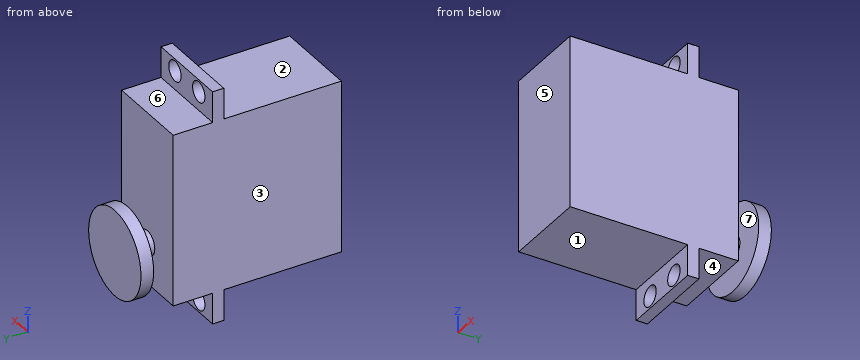
```python
from build123d import *

# Parameters (mm, degrees)
SKETCH1_W           = 19.8
SKETCH1_H           = 40.15
BOSS_EXTRUDE1_DEPTH = 39.2
SKETCH4_W           = 19.8
SKETCH4_H           = 2.6
BOSS_EXTRUDE2_DEPTH = 7.225
CUT_EXTRUDE1_REACH  = 43.753
SKETCH5_R           = 2.375
SKETCH6_R           = 2.825
BOSS_EXTRUDE3_DEPTH = 4.65
SKETCH8_R           = 10.05
BOSS_EXTRUDE4_DEPTH = 2.95


with BuildPart() as part:
    # Sketch1 → Boss-Extrude1 (new body)
    with BuildSketch(Plane(origin=(0, 0, 0), x_dir=(1, 0, 0), z_dir=(0, 1, 0))):
        Rectangle(SKETCH1_W, SKETCH1_H)
    extrude(amount=BOSS_EXTRUDE1_DEPTH)

    # Sketch4 → Boss-Extrude2 (add)
    with BuildSketch(Plane(origin=(0, 0, -20.075), x_dir=(-1, 0, 0), z_dir=(0, 0, -1))):
        with Locations((0, 28.7)):
            Rectangle(SKETCH4_W, SKETCH4_H)
    boss_extrude2 = extrude(amount=BOSS_EXTRUDE2_DEPTH)

    # Sketch5 → Cut-Extrude1 (cut, up to next)
    with BuildSketch(Plane(origin=(0, 30, 0), x_dir=(1, 0, 0), z_dir=(0, 1, 0)), mode=Mode.PRIVATE) as cut_extrude1_sk1:
        with Locations(Location((4.575, 24.45, 0), (0, 0, 270))):
            Circle(SKETCH5_R)
    cut_extrude1_tool1 = extrude(cut_extrude1_sk1.sketch, amount=-CUT_EXTRUDE1_REACH, mode=Mode.PRIVATE) & part.part
    # Sketch5 → Cut-Extrude1 (cut, up to next)
    with BuildSketch(Plane(origin=(0, 30, 0), x_dir=(1, 0, 0), z_dir=(0, 1, 0)), mode=Mode.PRIVATE) as cut_extrude1_sk2:
        with Locations(Location((-4.575, 24.45, 0), (0, 0, 270))):
            Circle(SKETCH5_R)
    cut_extrude1_tool2 = extrude(cut_extrude1_sk2.sketch, amount=-CUT_EXTRUDE1_REACH, mode=Mode.PRIVATE) & part.part
    cut_extrude1_1 = cut_extrude1_tool1.solids().sort_by_distance((4.575, 30, -24.45))[0]
    add(cut_extrude1_1, mode=Mode.SUBTRACT)
    cut_extrude1_2 = cut_extrude1_tool2.solids().sort_by_distance((-4.575, 30, -24.45))[0]
    add(cut_extrude1_2, mode=Mode.SUBTRACT)
    cut_extrude1 = cut_extrude1_1 + cut_extrude1_2  # Cut-Extrude1 as one shape, for the pattern or mirror that repeats it

    # Mirror2: Boss-Extrude2, Cut-Extrude1 across plane
    add(boss_extrude2.mirror(Plane.XY))
    add(cut_extrude1.mirror(Plane.XY), mode=Mode.SUBTRACT)

    # Sketch6 → Boss-Extrude3 (add)
    with BuildSketch(Plane(origin=(0, 39.2, 0), x_dir=(1, 0, 0), z_dir=(0, 1, 0))):
        with Locations(Location((0, 10.475, 0), (0, 0, 270))):
            Circle(SKETCH6_R)
    extrude(amount=BOSS_EXTRUDE3_DEPTH)

    # Sketch8 → Boss-Extrude4 (add)
    with BuildSketch(Plane(origin=(0, 43.85, 0), x_dir=(1, 0, 0), z_dir=(0, 1, 0))):
        with Locations(Location((0, 10.475, 0), (0, 0, 270))):
            Circle(SKETCH8_R)
    extrude(amount=BOSS_EXTRUDE4_DEPTH)


solid = part.part
```
Build history of the part. All positions in model axes, mm. Face numbers are marked on the shaded views. A direction names the side the tool comes from. Give positions to 0.01 mm unless a question says otherwise; leave off trailing zeros. Loops run counter-clockwise (first coordinate to the right, second up) from the corner with the lowest first, then second, coordinate; pieces in that order, holes last. Notation, with made-up numbers: (17, 23.25) - (43, 23.25) arc R27 ccw to (43, 47.25) - close; hole circle Ø8 at (-18.75, -30). An arc over 180 degrees is marked (long way). Use a Markdown table: item, result.
(1) Wall check: line 1 along X through (y, z) = (28.9, -24.45); line 2 along Z through (x, y) = (-5.25, 29.5); line 3 along Y through (x, z) = (4.5, -16). Give the ranges that are in metal, low to high.
Taken from the geometry:
| item | result |
|---|---|
| line 1 | -9.9 to -6.95, -2.2 to 2.2, 6.95 to 9.9 |
| line 2 | -27.3 to -26.73, -22.17 to 22.17, 26.73 to 27.3 |
| line 3 | 0 to 39.2, 43.85 to 46.8 |
(2) Band-saw the part on D-D (x = 0). Give the cut face in (y, z) (3 decimals), and give its area (3 significant figures).
Taken from the geometry:
| item | result |
|---|---|
| outline | (0, -20.075) - (27.4, -20.075) - (27.4, -27.3) - (30, -27.3) - (30, -20.075) - (39.2, -20.075) - (39.2, -13.3) - (43.85, -13.3) - (43.85, -20.525) - (46.8, -20.525) - (46.8, -0.425) - (43.85, -0.425) - (43.85, -7.65) - (39.2, -7.65) - (39.2, 20.075) - (30, 20.075) - (30, 27.3) - (27.4, 27.3) - (27.4, 20.075) - (0, 20.075) - close |
| area | 1,700 mm2 |
(3) Band-saw the part on A-A (z = 24.45). Give the cut face in (x, y).
Taken from the geometry:
| item | result |
|---|---|
| outline | (-9.9, 27.4) - (-6.95, 27.4) - (-6.95, 30) - (-9.9, 30) - close; (-2.2, 27.4) - (2.2, 27.4) - (2.2, 30) - (-2.2, 30) - close; (6.95, 27.4) - (9.9, 27.4) - (9.9, 30) - (6.95, 30) - close |
(4) Drop flat-ended pins along their axis: pin 1 Ø19.5 at (y, z) = (18.5, -2) entering from -X; pin 2 Ø6 at (x, z) = (4.575, 24.45) entering from -Y; pin 3 Ø5 at (y, z) = (30.5, 3.5) entering from +X; pin 4 Ø4.5 at (x, z) = (-4.575, 24.45) entering from -Y. Give the stop position or say it passes through.
Taken from the geometry:
| item | result |
|---|---|
| pin 1 | x = -9.9 |
| pin 2 | y = 27.4 |
| pin 3 | x = 9.9 |
| pin 4 | through |
(5) Which spindle directions (+Z, -Z, +X, -X, +Y, -Y) get a long thin tool onto all of the face, cutting with end or side? Do the marked faces 1, 2, 3 and 4. Say none if no direction does.
Taken from the geometry:
| item | result |
|---|---|
| face 1 | -Z, +X, -X, -Y |
| face 2 | +Z, +X, -X, -Y |
| face 3 | +Z, -Z, -X, -Y |
| face 4 | -Z, +X, -X |
(6) Band-saw the part on B-B (x = 7.75). Give the cut face in (y, z) (3 decimals), and give its area (3 significant figures).
Taken from the geometry:
| item | result |
|---|---|
| outline | (0, -20.075) - (27.4, -20.075) - (27.4, -27.3) - (30, -27.3) - (30, -20.075) - (39.2, -20.075) - (39.2, 20.075) - (30, 20.075) - (30, 27.3) - (27.4, 27.3) - (27.4, 20.075) - (0, 20.075) - close; (43.85, -16.873) - (46.8, -16.873) - (46.8, -4.077) - (43.85, -4.077) - close |
| area | 1,650 mm2 |
(7) Band-saw the part on C-C (x = 3.5). Give the cut face in (y, z) (3 decimals), and give its area (3 significant figures).
Taken from the geometry:
| item | result |
|---|---|
| outline | (0, -20.075) - (27.4, -20.075) - (27.4, -22.332) - (30, -22.332) - (30, -20.075) - (39.2, -20.075) - (39.2, 20.075) - (30, 20.075) - (30, 22.332) - (27.4, 22.332) - (27.4, 20.075) - (0, 20.075) - close; (27.4, -27.3) - (30, -27.3) - (30, -26.568) - (27.4, -26.568) - close; (27.4, 26.568) - (30, 26.568) - (30, 27.3) - (27.4, 27.3) - close; (43.85, -19.896) - (46.8, -19.896) - (46.8, -1.054) - (43.85, -1.054) - close |
| area | 1,650 mm2 |
(8) Pull direction Y, two halves, no side cores. Call the marked faces 5, 6 and 7: +Y half, -Y half, draft (parallel to the pull), parting line (faces both ways), or undercut.
Taken from the geometry:
| item | result |
|---|---|
| face 5 | -Y half |
| face 6 | draft |
| face 7 | undercut |
